```python
from build123d import *

# Parameters (mm, degrees)
SKETCH2_W           = 85
SKETCH2_H           = 50
BOSS_EXTRUDE2_DEPTH = 5
SKETCH3_R           = 17.0688374
SKETCH3_R_2         = 8
BOSS_EXTRUDE4_DEPTH = 50
SKETCH5_R           = 1.5
CUT_EXTRUDE1_DEPTH  = 50


with BuildPart() as part:
    # Sketch2 → Boss-Extrude2 (new body)
    with BuildSketch(Plane(origin=(0, 0, 0), x_dir=(1, 0, 0), z_dir=(0, 1, 0))):
        with Locations((42.5, 25)):
            Rectangle(SKETCH2_W, SKETCH2_H)
    extrude(amount=BOSS_EXTRUDE2_DEPTH)

    # Sketch3 → Boss-Extrude4 (add)
    with BuildSketch(Plane.XY):
        with Locations((42.5, 17.131570827)):
            Circle(SKETCH3_R)
        with Locations((42.5, 17.131570827)):
            Circle(SKETCH3_R_2, mode=Mode.SUBTRACT)
    extrude(amount=-BOSS_EXTRUDE4_DEPTH)

    # Sketch5 → Cut-Extrude1 (cut)
    with BuildSketch(Plane(origin=(0, 5, 0), x_dir=(1, 0, 0), z_dir=(0, 1, 0))):
        with Locations(Location((11.665290462, 36.170405123, 0), (0, 0, 270))):
            Circle(SKETCH5_R)
    extrude(amount=-CUT_EXTRUDE1_DEPTH, mode=Mode.SUBTRACT)


solid = part.part
```
CAD build for the part. Positions are in the model's coordinates, mm. A direction names the side the tool comes from. Give positions to 0.01 mm unless a question says otherwise; leave off trailing zeros. Write each loop counter-clockwise with the first axis right and the second up, starting at its lowest first coordinate (ties: lowest second). Pieces come first, ordered by that corner, then holes. Notation, with made-up numbers: M -39,67.5 L -15,67.5 A19 cw -15,99.5 Z; hole C 59,-12 d1. An arc over 180 degrees is marked long. Return JSON: item names as keys, results as strings. Group by question number.
(1) Band-saw the part on B-B (y = 12). Give the cut face in (x, z).
(2) Band-saw the part on D-D (x = 64.5). Give the cut face in (y, z).
(3) Band-saw the part on A-A (x = 42.5). Give the cut face in (y, z), and give its area (3 significant figures).
(4) Mould opens along Z. For faces 3 (the face through (36.604, 22.538, -24.65)), 4 (the face through (42, 8, 0)), 5 (the face through (42, 8, -50)), 6 (the face through (11.091, 2.535, -34.785)) say: pulls with the +Z half, pulls with the -Z half, needs draft (parallel to the pull), parting line crosses it, or undercut.
(5) 3-axis set-ups, long thin cutter, end or side, ignore diameter. For faces 1 (the face through (70, 5, -25)), 2 (the face through (42, 0, -25)): which of +Z, -Z, +X, -X, +Y, -Y reach the whole face in a straight line?
(6) Band-saw the part on C-C (z = -19.5). Give the cut face in (x, y).
(7) Flat gauge pins, fed straight in: pin 1 Ø3 at (x, y) = (49, 18.5) entering from -Z; pin 2 Ø3 at (y, z) = (7.5, -29) entering from -X; pin 3 Ø4 at (x, z) = (8.5, -41) entering from +Y; pin 4 Ø3 at (x, z) = (37.5, -40.5) entering from +Y. Where does each tip first touch, or does it go through?
(8) Drill centre lines: L1, parallel to Y at x = 13.5, z = -10; L2, parallel to X at y = 10, z = -31.5; L3, parallel to X at y = 23, z = -33. Where is each one in solid material? Low to high. Write a range as [from, to].
Entries:
{
 "1": {"outline": "M 26.22,-50 L 36.36,-50 L 36.36,0 L 26.22,0 Z; M 48.64,-50 L 58.78,-50 L 58.78,0 L 48.64,0 Z"},
 "2": {"outline": "M 0,-50 L 5,-50 L 5,0 L 0,0 Z"},
 "3": {"outline": "M 0,-50 L 9.13,-50 L 9.13,0 L 0,0 Z; M 25.13,-50 L 34.2,-50 L 34.2,0 L 25.13,0 Z", "area": "910 mm^2"},
 "4": {"face 3": "needs draft", "face 4": "pulls with the +Z half", "face 5": "pulls with the -Z half", "face 6": "undercut"},
 "5": {"face 1": "+Z, -Z, +X", "face 2": "+Z, -Z, +X, -X, -Y"},
 "6": {"outline": "M 0,0 L 85,0 L 85,5 L 54.51,5 A17.07 ccw long 30.49,5 L 0,5 Z; hole C 42.5,17.13 d16"},
 "7": {"pin 1": "stops at z = -50", "pin 2": "stops at x = 27.49", "pin 3": "stops at y = 5", "pin 4": "stops at y = 33.84"},
 "8": {"L1": "y = [0, 5]", "L2": "x = [26.99, 38.87], [46.13, 58.01]", "L3": "x = [26.47, 37.06], [47.94, 58.53]"}
}
